The listing builds one solid part. Answer for the finished solid, in the listing's coordinates (mm). A direction names the side the tool comes from. Coordinates: 2 decimals unless noted, no trailing zeros. Write each loop counter-clockwise with the first axis right and the second up, starting at its lowest first coordinate (ties: lowest second). Pieces come first, ordered by that corner, then holes. Notation, with made-up numbers: M 37.5,68.5 L 85.5,68.5 A22 cw 85.5,104.5 Z; hole C 22,75.25 d1. An arc over 180 degrees is marked long. Put each result on its own line as item: value. Start each with the question number.
```python
from build123d import *

# Parameters (mm, degrees)
SKETCH1_W           = 30
SKETCH1_H           = 10.4
BOSS_EXTRUDE1_DEPTH = 2
SKETCH2_W           = 22
SKETCH2_H           = 6.4
CUT_EXTRUDE1_DEPTH  = 3
SKETCH4_W           = 30
SKETCH4_H           = 2
BOSS_EXTRUDE2_DEPTH = 45
SKETCH5_W           = 26
SKETCH5_H           = 26
CUT_EXTRUDE3_DEPTH  = 11.4
SKETCH6_W           = 26
SKETCH6_H           = 13
CUT_EXTRUDE4_DEPTH  = 11.4


with BuildPart() as part:
    # Sketch1 → Boss-Extrude1 (new body)
    with BuildSketch(Plane(origin=(0, 0, 0), x_dir=(1, 0, 0), z_dir=(0, 1, 0))):
        with Locations((15, -5.2)):
            Rectangle(SKETCH1_W, SKETCH1_H)
    extrude(amount=BOSS_EXTRUDE1_DEPTH)

    # Sketch2 → Cut-Extrude1 (cut, through all)
    with BuildSketch(Plane(origin=(0, 2, 0), x_dir=(1, 0, 0), z_dir=(0, 1, 0))):
        with Locations((15, -5.2)):
            Rectangle(SKETCH2_W, SKETCH2_H)
    extrude(amount=-CUT_EXTRUDE1_DEPTH, mode=Mode.SUBTRACT)

    # Sketch4 → Boss-Extrude2 (add)
    with BuildSketch(Plane(origin=(0, 2, 0), x_dir=(1, 0, 0), z_dir=(0, 1, 0))):
        with Locations((15, -1)):
            Rectangle(SKETCH4_W, SKETCH4_H)
    extrude(amount=-BOSS_EXTRUDE2_DEPTH)

    # Sketch5 → Cut-Extrude3 (cut, through all)
    with BuildSketch(Plane(origin=(0, 0, 0), x_dir=(-1, 0, 0), z_dir=(0, 0, -1))):
        with Locations((-15, -28)):
            Rectangle(SKETCH5_W, SKETCH5_H)
    extrude(amount=-CUT_EXTRUDE3_DEPTH, mode=Mode.SUBTRACT)

    # Sketch6 → Cut-Extrude4 (cut, through all)
    with BuildSketch(Plane(origin=(0, 0, 0), x_dir=(-1, 0, 0), z_dir=(0, 0, -1))):
        with Locations((-15, -6.5)):
            Rectangle(SKETCH6_W, SKETCH6_H)
    extrude(amount=-CUT_EXTRUDE4_DEPTH, mode=Mode.SUBTRACT)


solid = part.part
```
1) Given pin 1 Ø15 at (x, y) = (20, -31.5) entering from +Z; pin 2 Ø1 at (x, y) = (9, -14.5) entering from +Z, each flat-ended and moving along its own axis, determine where each tip first touches the part or whether it passes through.
2) A cutting plane is placed at A-A on y = -19. Write down the section's boundary in (x, z).
3) Determine the mould class of faces 1 (the face through (15, 1, 2)), 2 (the face through (15, -13, 1)), 3 (the face through (15, 2, 9)), 4 (the face through (2, -28, 1)) for opening direction Y: +Y half, -Y half, draft (parallel to the pull), parting line (faces both ways), or undercut.
4) A cutting plane is placed at C-C on z = 7.75. Write down the section's boundary in (x, y), then the cut area to 3 significant figures.
5) For faces 5 (the face through (4, 1, 5)), 6 (the face through (15, -41, 1)), 7 (the face through (15, 0, 9)), determine the directions among +Z, -Z, +X, -X, +Y, -Y from which every point of the face is accessible in a straight line to the end or side of a thin tool.
6) A cutting plane is placed at D-D on x = 11.5. Write down the section's boundary in (y, z).
7) A cutting plane is placed at B-B on x = 3. Write down the section's boundary in (y, z).
8) Straight lines are drawn through the part: probe 1 along Y at (x, z) = (10.5, 1.5); probe 2 along X at (y, z) = (-21.5, 0.75); probe 3 along Y at (x, z) = (1.25, 2.5). For each, find the intervals that lie inside material, in ascending order.
Answers follow:
1. pin 1: passes through
1. pin 2: stops at z = 2
2. outline: M 0,0 L 2,0 L 2,2 L 0,2 Z; M 28,0 L 30,0 L 30,2 L 28,2 Z
3. face 1: draft
3. face 2: undercut
3. face 3: +Y half
3. face 4: undercut
4. outline: M 0,0 L 4,0 L 4,2 L 0,2 Z; M 26,0 L 30,0 L 30,2 L 26,2 Z
4. area: 16.0 mm²
5. face 5: +Y, -Y
5. face 6: +Z, -Z
5. face 7: +Z
6. outline: M -43,0 L -41,0 L -41,2 L -43,2 Z; M -15,0 L -13,0 L -13,2 L -15,2 Z; M 0,0 L 2,0 L 2,2 L 0,2 Z; M 0,8.4 L 2,8.4 L 2,10.4 L 0,10.4 Z
7. outline: M -43,0 L -41,0 L -41,2 L -43,2 Z; M -15,0 L -13,0 L -13,2 L -15,2 Z; M 0,0 L 2,0 L 2,10.4 L 0,10.4 Z
8. probe 1: y = -43 to -41, -15 to -13, 0 to 2
8. probe 2: x = 0 to 2, 28 to 30
8. probe 3: y = 0 to 2
